Answer from the drawing. Dimensions are ordinates in mm from the lowest x, y and z of the part. Round coordinates to 2 decimals unless told otherwise and drop trailing zeros. Loops run counter-clockwise (first coordinate to the right, second up) from the corner with the lowest first, then second, coordinate; pieces in that order, holes last. Notation, with made-up numbers: (42, 7) - (66, 7) arc R25 ccw to (66, 33) - close; hole circle Ø10 at (43, 37). An arc over 180 degrees is marked (long way). Answer as CSV lines item,"result". Start each with the question number.
Q1. Straight lines are drawn through the part: L1, parallel to X at y = 29.5, z = 0.9; L2, parallel to Y at x = 59, z = 1.1; L3, parallel to Y at x = 49, z = 1.1. For each, find the intervals that lie inside material, in ascending order. Write a range as [from, to].
Q2. Section B-B on x = 49 is taken. Write down the section's boundary in (y, z), then the cut area to 3 significant figures.
Q3. Each of these flat-tipped pins is pushed along its axis until it touches: pin 1 Ø8 at (x, y) = (51, 19.5) entering from -Z; pin 2 Ø2.5 at (x, y) = (59, 7.5) entering from +Z. Where does it stop, or does it pass through?
Q4. Section A-A on y = 7.5 is taken. Write down the section's boundary in (x, z), then the cut area to 3 significant figures.
Q5. Section C-C on y = 45 is taken. Write down the section's boundary in (x, z), then the cut area to 4 significant figures.
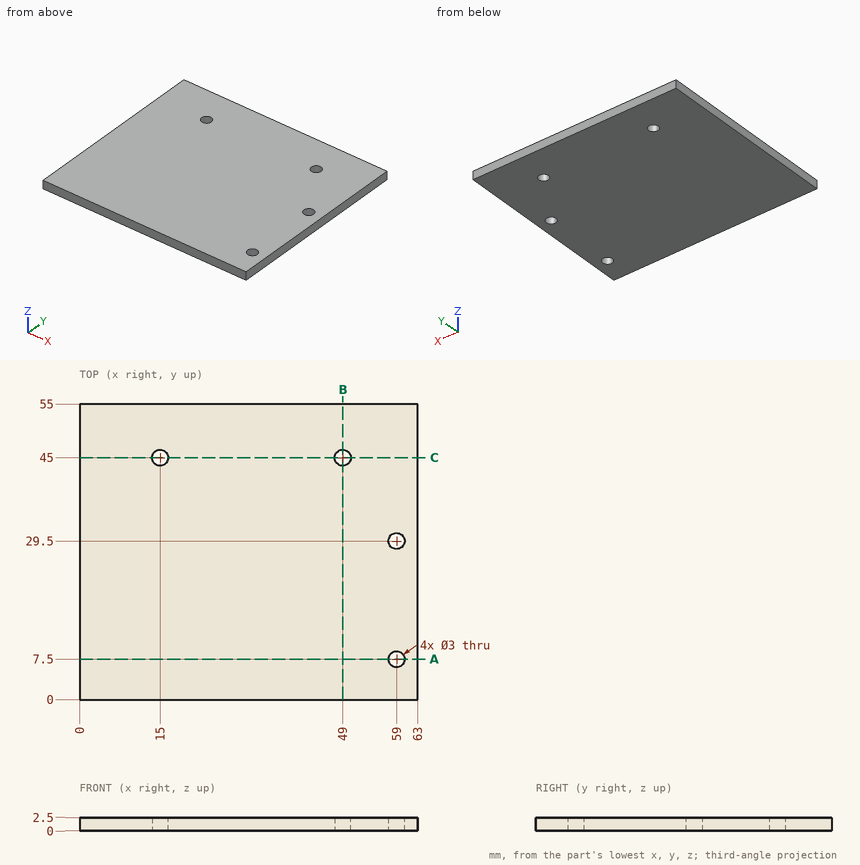
Findings:
1,L1,"x = [0, 57.5], [60.5, 63]"
1,L2,"y = [0, 6], [9, 28], [31, 55]"
1,L3,"y = [0, 43.5], [46.5, 55]"
2,outline,"(0, 0) - (43.5, 0) - (43.5, 2.5) - (0, 2.5) - close; (46.5, 0) - (55, 0) - (55, 2.5) - (46.5, 2.5) - close"
2,area,"130 mm^2"
3,pin 1,"stops at z = 0"
3,pin 2,"passes through"
4,outline,"(0, 0) - (57.5, 0) - (57.5, 2.5) - (0, 2.5) - close; (60.5, 0) - (63, 0) - (63, 2.5) - (60.5, 2.5) - close"
4,area,"150 mm^2"
5,outline,"(0, 0) - (13.5, 0) - (13.5, 2.5) - (0, 2.5) - close; (16.5, 0) - (47.5, 0) - (47.5, 2.5) - (16.5, 2.5) - close; (50.5, 0) - (63, 0) - (63, 2.5) - (50.5, 2.5) - close"
5,area,"142.5 mm^2"
